Geometry check sheet. Reference: the model listing, model coordinates, mm. Face numbers are marked on the shaded views. Give positions to 0.01 mm unless a question says otherwise; leave off trailing zeros. Write each loop counter-clockwise with the first axis right and the second up, starting at its lowest first coordinate (ties: lowest second). Pieces come first, ordered by that corner, then holes. Notation, with made-up numbers: (-9.75, 38) - (22.25, 38) arc R15 cw to (22.25, 57) - close; hole circle Ø5 at (88, 0). An arc over 180 degrees is marked (long way). Use a Markdown table: item, result.
```python
from build123d import *

# Parameters (mm, degrees)
SKETCH1_W             = 25.4
SKETCH1_H             = 25.4
SKETCH1_W_2           = 22.225
SKETCH1_H_2           = 22.225
EXTRUDE_THIN1_DEPTH   = 152.4
BOSS_EXTRUDE1_DEPTH   = 1.5875
BOSS_EXTRUDE2_START   = 22.225
BOSS_EXTRUDE2_DEPTH   = 1.5875
F_4_CLEARANCE_HOLE1_D = 3.2639
SKETCH11_R            = 6.35
BOSS_EXTRUDE3_DEPTH   = 1.5875
BOSS_EXTRUDE4_START   = -25.4
SKETCH11_3_R          = 6.35
BOSS_EXTRUDE4_DEPTH   = 1.5875


# Read off the part's stored shape, not the designer's step: Boss-Extrude2
with BuildPart() as part:
    # Sketch1 → Extrude-Thin1 (new, symmetric)
    with BuildSketch(Plane(origin=(0, 0, 0), x_dir=(1, 0, 0), z_dir=(0, 1, 0))):
        Rectangle(SKETCH1_W, SKETCH1_H)
        Rectangle(SKETCH1_W_2, SKETCH1_H_2, mode=Mode.SUBTRACT)
    extrude(amount=EXTRUDE_THIN1_DEPTH, both=True)

    # Sketch3 → Boss-Extrude1 (add)
    with BuildSketch(Plane(origin=(-11.1125, 0, 0), x_dir=(0, 0, -1), z_dir=(1, 0, 0))):
        with BuildLine():
            ThreePointArc((12.7, -161.925), (15.669940551, -159.872532015), (14.800065103, -156.36875))
            ThreePointArc((14.800065103, -156.36875), (13.387535234, -154.576190551), (12.7, -152.4))
            Line((12.7, -152.4), (-12.7, -152.4))
            ThreePointArc((-12.7, -152.4), (-13.387535234, -154.576190551), (-14.800065103, -156.36875))
            ThreePointArc((-14.800065103, -156.36875), (-15.669940551, -159.872532015), (-12.7, -161.925))
            Line((-12.7, -161.925), (12.7, -161.925))
        make_face()
    extrude(amount=-BOSS_EXTRUDE1_DEPTH)

    # Boss-Extrude2 outline → Boss-Extrude2 (add)
    with BuildSketch(Plane(origin=(-11.1125, 0, 0), x_dir=(0, 0, -1), z_dir=(1, 0, 0)).offset(BOSS_EXTRUDE2_START)):
        with BuildLine():
            Line((-12.7, -161.925), (12.7, -161.925))
            ThreePointArc((12.7, -161.925), (15.669940551, -159.872532015), (14.800065103, -156.36875))
            ThreePointArc((14.800065103, -156.36875), (13.387535234, -154.576190551), (12.7, -152.4))
            Line((12.7, -152.4), (-12.7, -152.4))
            ThreePointArc((-12.7, -152.4), (-13.387535234, -154.576190551), (-14.800065103, -156.36875))
            ThreePointArc((-14.800065103, -156.36875), (-15.669940551, -159.872532015), (-12.7, -161.925))
        make_face()
    extrude(amount=BOSS_EXTRUDE2_DEPTH)

    # #4 Clearance Hole1 (through all)
    with Locations(Plane.ZY.offset(12.7)):
        with Locations((-12.7, -158.75), (12.7, -158.75)):
            Hole(F_4_CLEARANCE_HOLE1_D / 2)

    # Sketch11 → Boss-Extrude3 (add)
    with BuildSketch(Plane.ZY.offset(12.7)):
        with Locations((-6.35, 165.1)):
            Circle(SKETCH11_R)
        with BuildLine():
            Line((10.840128061, 156.890128061), (-1.859871939, 169.590128061))
            ThreePointArc((-1.859871939, 169.590128061), (-0.483364969, 167.530039796), (0, 165.1))
            ThreePointArc((0, 165.1), (-6.35, 158.75), (-12.7, 165.1))
            Line((-12.7, 165.1), (-12.7, 152.4))
            Line((-12.7, 152.4), (12.7, 152.4))
            ThreePointArc((12.7, 152.4), (12.216635031, 154.830039796), (10.840128061, 156.890128061))
        make_face()
    extrude(amount=-BOSS_EXTRUDE3_DEPTH)

    # Sketch11<3> → Boss-Extrude4 (add)
    with BuildSketch(Plane.ZY.offset(12.7).offset(BOSS_EXTRUDE4_START)):
        with BuildLine():
            Line((10.840128061, 156.890128061), (-1.859871939, 169.590128061))
            ThreePointArc((-1.859871939, 169.590128061), (-0.483364969, 167.530039796), (0, 165.1))
            ThreePointArc((0, 165.1), (-6.35, 158.75), (-12.7, 165.1))
            Line((-12.7, 165.1), (-12.7, 152.4))
            Line((-12.7, 152.4), (12.7, 152.4))
            ThreePointArc((12.7, 152.4), (12.216635031, 154.830039796), (10.840128061, 156.890128061))
        make_face()
        with Locations((-6.35, 165.1)):
            Circle(SKETCH11_3_R)
    extrude(amount=BOSS_EXTRUDE4_DEPTH)


solid = part.part
```
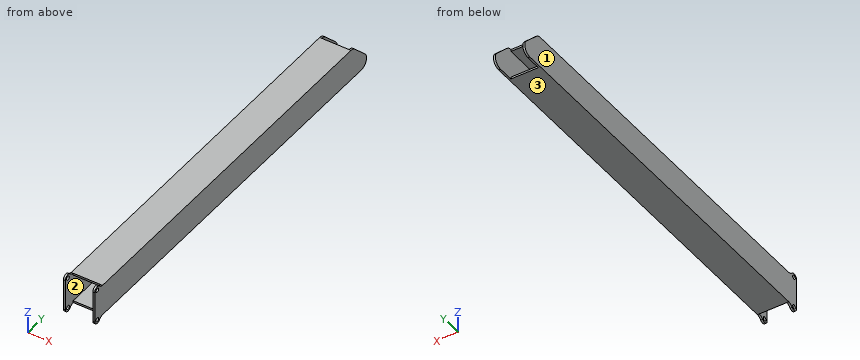
1) Section check B-B on y = 59.5. Record the boundary of the cut face in (x, z), then the cut area to 3 significant figures.
Working result:
| item | result |
|---|---|
| outline | (-12.7, -12.7) - (12.7, -12.7) - (12.7, 12.7) - (-12.7, 12.7) - close; hole (-11.11, -11.11) - (11.11, -11.11) - (11.11, 11.11) - (-11.11, 11.11) - close |
| area | 151 mm² |
2) Section check A-A on x = 2.25. Record the boundary of the cut face in (y, z).
Working result:
| item | result |
|---|---|
| outline | (-152.4, -12.7) - (152.4, -12.7) - (152.4, -11.11) - (-152.4, -11.11) - close; (-152.4, 11.11) - (152.4, 11.11) - (152.4, 12.7) - (-152.4, 12.7) - close |
3) Section check C-C on z = 1.5. Record the boundary of the cut face in (x, y) (1 decimal).
Working result:
| item | result |
|---|---|
| outline | (-12.7, -161.9) - (-11.1, -161.9) - (-11.1, 166.2) - (-12.7, 166.2) - close; (11.1, -161.9) - (12.7, -161.9) - (12.7, 166.2) - (11.1, 166.2) - close |
4) Material ranges on L1, parallel to Z at x = -12.25, y = -158.75 (3 decimals); L2, parallel to Z at x = 6.25, y = -69.5, recorded low to high. Write a range as from..to.
Working result:
| item | result |
|---|---|
| L1 | z = -15.875..-14.332, -11.068..11.068, 14.332..15.875 |
| L2 | z = -12.7..-11.11, 11.11..12.7 |
5) Mould release check, pull along Z, two halves, no side actions. Record for the marked faces 1, 2 and 3: pulls with the +Z half, pulls with the -Z half, needs draft (parallel to the pull), parting line crosses it, or undercut.
Working result:
| item | result |
|---|---|
| face 1 | needs draft |
| face 2 | undercut |
| face 3 | pulls with the -Z half |
6) Depth check by flat-ended pin: P1, Ø2, axis at x = -8.5, y = 52.5, coming from the -Z side; P2, Ø0.8, axis at x = -2, z = 12, coming from the -Y side; P3, Ø1.3, axis at x = 4.5, z = 12, coming from the +Y side. Enter the tip coordinate at first touch or a pass-through.
Working result:
| item | result |
|---|---|
| P1 | stops at z = -12.7 |
| P2 | stops at y = -152.4 |
| P3 | stops at y = 152.4 |
